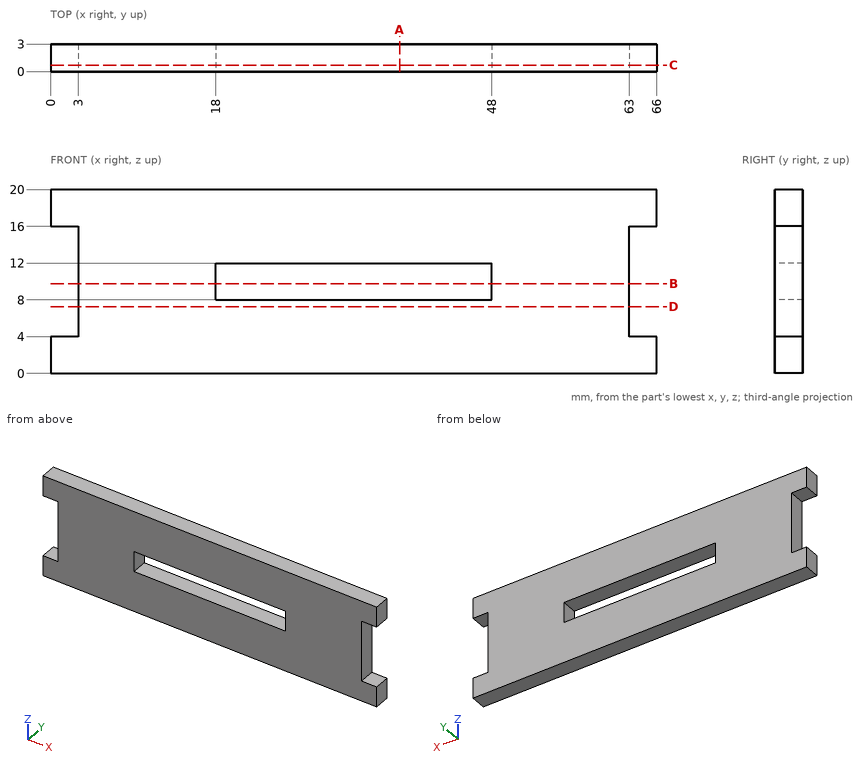
Verification items for this drawing (mm, ordinates from the low corner). Coordinates: 2 decimals unless noted, no trailing zeros. Order: outer loops, then holes, each group sorted by start corner. A loop starts at its lowest first (then second) coordinate and runs counter-clockwise, first axis right, second up. Notation, with made-up numbers: M 39.25,78 L 81.25,78 A18 ccw 81.25,92 Z; hole C 83,-23.75 d10. An arc over 180 degrees is marked long. One line per item, written item: value. Start each with the question number.
Item 1: Thickness scan on probe 1 along X at (y, z) = (0.35, 9.5); probe 2 along Z at (x, y) = (45.5, 0.75); probe 3 along X at (y, z) = (1.6, 13.75). Record the ranges inside material, lowest first.
Item 2: Depth check by flat-ended pin: P1, Ø1, axis at y = 2, z = 11.5, coming from the -X side; P2, Ø0.9, axis at y = 1.5, z = 10.5, coming from the +X side. Enter the tip coordinate at first touch or a pass-through.
Item 3: Sectioned sample at C-C on y = 0.7. Record the cut outline in (x, z).
Item 4: Sectioned sample at D-D on z = 7.25. Record the cut outline in (x, y).
Item 5: Sectioned sample at B-B on z = 9.75. Record the cut outline in (x, y), then the cut area to 3 significant figures.
Item 6: Sectioned sample at A-A on x = 38. Record the cut outline in (y, z).
Calculated:
1. probe 1: 3 to 18, 48 to 63
1. probe 2: 0 to 8, 12 to 20
1. probe 3: 3 to 63
2. P1: x = 3
2. P2: x = 63
3. outline: M 0,0 L 66,0 L 66,4 L 63,4 L 63,16 L 66,16 L 66,20 L 0,20 L 0,16 L 3,16 L 3,4 L 0,4 Z; hole M 18,8 L 48,8 L 48,12 L 18,12 Z
4. outline: M 3,0 L 63,0 L 63,3 L 3,3 Z
5. outline: M 3,0 L 18,0 L 18,3 L 3,3 Z; M 48,0 L 63,0 L 63,3 L 48,3 Z
5. area: 90.0 mm^2
6. outline: M 0,0 L 3,0 L 3,8 L 0,8 Z; M 0,12 L 3,12 L 3,20 L 0,20 Z
